Check sheet for the modelled part. Datum: model origin and axes. Units: mm. A direction names the side the tool comes from. Give positions to 0.01 mm unless a question says otherwise; leave off trailing zeros. Order: outer loops, then holes, each group sorted by start corner. A loop starts at its lowest first (then second) coordinate and runs counter-clockwise, first axis right, second up.
from build123d import *

# Parameters (mm, degrees)
SKETCH1_R           = 57.5
SKETCH1_R_2         = 54.5
BOSS_EXTRUDE1_DEPTH = 120
SKETCH4_OUTSIDE_W   = 157.422
SKETCH4_OUTSIDE_H   = 157.422
CUT_EXTRUDE1_DEPTH  = 64
SKETCH5_OUTSIDE_W   = 157.422
SKETCH5_OUTSIDE_H   = 157.422
CUT_EXTRUDE2_DEPTH  = 30


with BuildPart() as part:
    # Sketch1 → Boss-Extrude1 (new body)
    with BuildSketch(Plane(origin=(0, 0, 0), x_dir=(1, 0, 0), z_dir=(0, 1, 0))):
        with Locations(Location((0, 0, 0), (0, 0, 270))):
            Circle(SKETCH1_R)
        with Locations(Location((0, 0, 0), (0, 0, 270))):
            Circle(SKETCH1_R_2, mode=Mode.SUBTRACT)
    extrude(amount=BOSS_EXTRUDE1_DEPTH)

    # Sketch4 outside → Cut-Extrude1 (cut)
    with BuildSketch(Plane(origin=(0, 120, 0), x_dir=(1, 0, 0), z_dir=(0, 1, 0))):
        Rectangle(SKETCH4_OUTSIDE_W, SKETCH4_OUTSIDE_H)
        with BuildLine():
            Line((-50.133042419, 28.158978281), (50.133042419, -28.158978281))
            ThreePointArc((50.133042419, -28.158978281), (-28.158978281, -50.133042419), (-50.133042419, 28.158978281))
        make_face(mode=Mode.SUBTRACT)
    extrude(amount=-CUT_EXTRUDE1_DEPTH, mode=Mode.SUBTRACT)

    # Sketch5 outside → Cut-Extrude2 (cut)
    with BuildSketch(Plane(origin=(0, 120, 0), x_dir=(1, 0, 0), z_dir=(0, 1, 0))):
        Rectangle(SKETCH5_OUTSIDE_W, SKETCH5_OUTSIDE_H)
        with BuildLine():
            Line((-56.185392762, -12.22504152), (18.796201116, -54.341078602))
            ThreePointArc((18.796201116, -54.341078602), (-28.158978281, -50.133042419), (-56.185392762, -12.22504152))
        make_face(mode=Mode.SUBTRACT)
    extrude(amount=-CUT_EXTRUDE2_DEPTH, mode=Mode.SUBTRACT)


solid = part.part
1) Depth check by flat-ended pin: pin 1 Ø4 at (x, y) = (-34, 51) entering from -Z; pin 2 Ø4 at (x, y) = (5.5, 73.5) entering from +Z; pin 3 Ø14 at (x, z) = (27, 42.5) entering from +Y. Enter the tip coordinate at first touch or a pass-through.
Recorded:
pin 1: stops at z = -47.77
pin 2: stops at z = 57.39
pin 3: stops at y = 90
2) Section check B-B, the plane z = 0. Record the cut outline in (x, y).
Recorded:
outline: (-57.5, 0) - (-54.5, 0) - (-54.5, 90) - (-57.5, 90) - close; (54.5, 0) - (57.5, 0) - (57.5, 56) - (54.5, 56) - close
3) Section check D-D, the plane y = 100.5. Record the cut outline in (x, z), then the cut area to 3 significant figures.
Recorded:
outline: (-56.19, 12.23) - (-52.61, 14.23) arc R54.5 cw to (15.22, 52.33) - (18.8, 54.34) arc R57.5 ccw to start
area: 276 mm2
4) Section check C-C, the plane y = 17. Record the cut outline in (x, z).
Recorded:
outline: circle Ø115 at (0, 0); hole circle Ø109 at (0, 0)
5) Material ranges on L1, parallel to X at y = 32, z = 0; L2, parallel to Z at x = 0, y = 64, recorded low to high.
Recorded:
L1: x = -57.5 to -54.5, 54.5 to 57.5
L2: z = 54.5 to 57.5
6) Set-up check for faces 1 (the face through (-54.422, 105.21, 13.216)), 2 (the face through (-22.023, 45.827, 53.115)): record each of +Z, -Z, +X, -X, +Y, -Y from which the full face is reachable in a straight line by a thin tool's end or side.
Recorded:
face 1: -Z, +X, +Y
face 2: +Y, -Y
7) Section check A-A, the plane x = 0. Record the cut outline in (y, z), then the cut area to 3 significant figures.
Recorded:
outline: (0, -57.5) - (56, -57.5) - (56, -54.5) - (0, -54.5) - close; (0, 54.5) - (120, 54.5) - (120, 57.5) - (0, 57.5) - close
area: 528 mm2
8) Draft check along X on faces 3 (the face through (-20.874, 45.827, 50.344)), 4 (the face through (16.98, 105.21, 53.32)), 5 (the face through (23, 56, -50)). Enter one of: +X half, -X half, draft (parallel to the pull), parting line (faces both ways), or undercut.
Recorded:
face 3: undercut
face 4: +X half
face 5: draft
